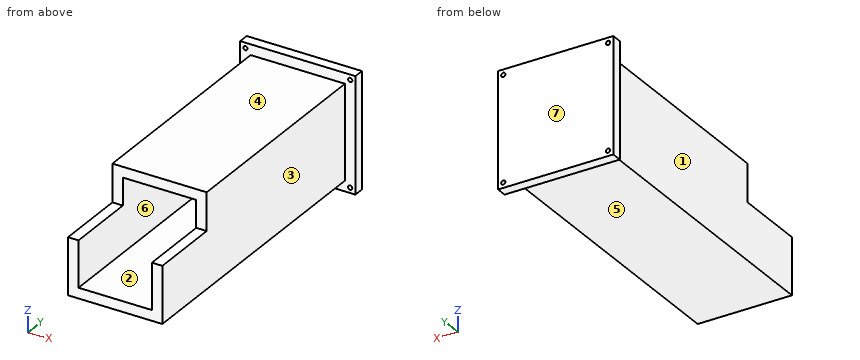
```python
from build123d import *

# Parameters (mm, degrees)
CROQUIS1_W                 = 45
CROQUIS1_H                 = 45
SALIENTE_EXTRUIR1_DEPTH    = 300
CROQUIS4_W                 = 18
CROQUIS4_H                 = 34
CORTAR_EXTRUIR2_DEPTH      = 46
CROQUIS8_W                 = 35
CROQUIS8_H                 = 35
CORTAR_EXTRUIR3_DEPTH      = 301
CROQUIS9_W                 = 35
CROQUIS9_H                 = 21.174410022
CORTAR_EXTRUIR4_DEPTH      = 10
CROQUIS10_R                = 1
CORTAR_EXTRUIR5_DEPTH      = 10
CROQUIS11_W                = 45
CROQUIS11_H                = 26.387879272
CORTAR_EXTRUIR6_DEPTH      = 46
CROQUIS13_W                = 45
CROQUIS13_H                = 133.61212073
CORTAR_EXTRUIR9_DEPTH      = 23.5
CORTAR_EXTRUIR9_DEPTH_BACK = 23.5
CROQUIS14_W                = 55
CROQUIS14_H                = 55
CROQUIS14_R                = 1
SALIENTE_EXTRUIR3_DEPTH    = 5


with BuildPart() as part:
    # Croquis1 → Saliente-Extruir1 (new body)
    with BuildSketch(Plane(origin=(0, 0, 0), x_dir=(1, 0, 0), z_dir=(0, 1, 0))):
        Rectangle(CROQUIS1_W, CROQUIS1_H)
    extrude(amount=SALIENTE_EXTRUIR1_DEPTH)

    # Croquis4 → Cortar-Extruir2 (cut, through all)
    with BuildSketch(Plane.ZY.offset(22.5)):
        with Locations((13.5, 17)):
            Rectangle(CROQUIS4_W, CROQUIS4_H)
    extrude(amount=-CORTAR_EXTRUIR2_DEPTH, mode=Mode.SUBTRACT)

    # Croquis8 → Cortar-Extruir3 (cut, through all)
    with BuildSketch(Plane(origin=(0, 300, 0), x_dir=(1, 0, 0), z_dir=(0, 1, 0))):
        Rectangle(CROQUIS8_W, CROQUIS8_H)
    extrude(amount=-CORTAR_EXTRUIR3_DEPTH, mode=Mode.SUBTRACT)

    # Croquis9 → Cortar-Extruir4 (cut)
    with BuildSketch(Plane(origin=(0, 0, -22.5), x_dir=(-1, 0, 0), z_dir=(0, 0, -1))):
        with Locations((0, 260)):
            Rectangle(CROQUIS9_W, CROQUIS9_H)
    extrude(amount=-CORTAR_EXTRUIR4_DEPTH, mode=Mode.SUBTRACT)

    # Croquis10 → Cortar-Extruir5 (cut)
    with BuildSketch(Plane.XY.offset(22.5)):
        with Locations((0, 260)):
            Circle(CROQUIS10_R)
    extrude(amount=-CORTAR_EXTRUIR5_DEPTH, mode=Mode.SUBTRACT)

    # Croquis11 → Cortar-Extruir6 (cut, through all)
    with BuildSketch(Plane.XY.offset(22.5)):
        with Locations((0, 286.806060364)):
            Rectangle(CROQUIS11_W, CROQUIS11_H)
    extrude(amount=-CORTAR_EXTRUIR6_DEPTH, mode=Mode.SUBTRACT)

    # Croquis13 → Cortar-Extruir9 (cut, two sides)
    with BuildSketch(Plane(origin=(0, 0, 0), x_dir=(0, 0, -1), z_dir=(1, 0, 0))) as cortar_extruir9_sk:
        with Locations((0, 206.806060363)):
            Rectangle(CROQUIS13_W, CROQUIS13_H)
    extrude(amount=CORTAR_EXTRUIR9_DEPTH, mode=Mode.SUBTRACT)
    extrude(cortar_extruir9_sk.sketch, amount=-CORTAR_EXTRUIR9_DEPTH_BACK, mode=Mode.SUBTRACT)

    # Croquis14 → Saliente-Extruir3 (add)
    with BuildSketch(Plane(origin=(0, 139.999999998, 0), x_dir=(1, 0, 0), z_dir=(0, 1, 0))):
        Rectangle(CROQUIS14_W, CROQUIS14_H)
        with Locations((-25, 25)):
            Circle(CROQUIS14_R, mode=Mode.SUBTRACT)
        with Locations((25, -25)):
            Circle(CROQUIS14_R, mode=Mode.SUBTRACT)
        with Locations((25, 25)):
            Circle(CROQUIS14_R, mode=Mode.SUBTRACT)
        with Locations((-25, -25)):
            Circle(CROQUIS14_R, mode=Mode.SUBTRACT)
    extrude(amount=SALIENTE_EXTRUIR3_DEPTH)


solid = part.part
```
Source: CAD feature listing. Evaluate the final solid. Frame: model axes, mm. Face numbers are marked on the shaded views. A direction names the side the tool comes from. Round coordinates to 2 decimals unless told otherwise and drop trailing zeros. Order: outer loops, then holes, each group sorted by start corner. A loop starts at its lowest first (then second) coordinate and runs counter-clockwise, first axis right, second up. Notation, with made-up numbers: (74, 30.5) -> (129, 30.5) arc R23 cw to (129, 42.5) -> close; hole circle Ø4 at (20.5, -4.5). An arc over 180 degrees is marked (long way). Use CSV: the item, a comma, the result in double quotes.
(1) Section C-C on z = -16. Return the cut outline in (x, y), and give its area (4 significant figures).
Report:
outline,"(-27.5, 140) -> (-22.5, 140) -> (-22.5, 0) -> (-17.5, 0) -> (-17.5, 140) -> (17.5, 140) -> (17.5, 0) -> (22.5, 0) -> (22.5, 140) -> (27.5, 140) -> (27.5, 145) -> (-27.5, 145) -> close"
area,"1,675 mm^2"
(2) Ray query, L1, parallel to X at y = 141, z = 25; L2, parallel to X at y = 110.5, z = -8. Return the intervals inside material, ascending.
Report:
L1,"-27.5 to -26, -24 to 24, 26 to 27.5"
L2,"-22.5 to -17.5, 17.5 to 22.5"
(3) Section A-A on y = 57. Return the cut outline in (x, z).
Report:
outline,"(-22.5, -22.5) -> (22.5, -22.5) -> (22.5, 22.5) -> (-22.5, 22.5) -> close; hole (-17.5, -17.5) -> (17.5, -17.5) -> (17.5, 17.5) -> (-17.5, 17.5) -> close"
(4) Access query for the marked faces 1, 2, 3 and 4. Directions: +Z, -Z, +X, -X, +Y, -Y. A direction counts if a zero-diameter tool reaches every point of the face in a straight line with its end or side. Return the directions, or none.
Report:
face 1,"+Z, -Z, -X, -Y"
face 2,"-Y"
face 3,"+Z, -Z, +X, -Y"
face 4,"+Z, +X, -X, -Y"
(5) Section D-D on x = -8. Return the cut outline in (y, z), and give its area (4 significant figures).
Report:
outline,"(0, -22.5) -> (140, -22.5) -> (140, -27.5) -> (145, -27.5) -> (145, 27.5) -> (140, 27.5) -> (140, 22.5) -> (34, 22.5) -> (34, 17.5) -> (140, 17.5) -> (140, -17.5) -> (0, -17.5) -> close"
area,"1,505 mm^2"
(6) Section B-B on x = 20.5. Return the cut outline in (y, z), and give its area (3 significant figures).
Report:
outline,"(0, -22.5) -> (140, -22.5) -> (140, -27.5) -> (145, -27.5) -> (145, 27.5) -> (140, 27.5) -> (140, 22.5) -> (34, 22.5) -> (34, 4.5) -> (0, 4.5) -> close"
area,"5,960 mm^2"
(7) Pull-direction query (Z, two-part tool) for the marked faces 5, 6 and 7; classes: +Z half, -Z half, draft (parallel to the pull), parting line (faces both ways), or undercut.
Report:
face 5,"-Z half"
face 6,"undercut"
face 7,"draft"
(8) First-contact query: pin 1 Ø4 at (y, z) = (96.5, 7) entering from -X; pin 2 Ø10 at (x, z) = (3.5, 10) entering from -Y; pin 3 Ø10.5 at (x, y) = (-5, 73) entering from -Z. Flat tips, straight axial feed; report the tip coordinate or a pass-through.
Report:
pin 1,"x = -22.5"
pin 2,"y = 140"
pin 3,"z = -22.5"
